Model file for the job. Use its own axes, mm. A direction names the side the tool comes from. Coordinates: 2 decimals unless noted, no trailing zeros. Order: outer loops, then holes, each group sorted by start corner. A loop starts at its lowest first (then second) coordinate and runs counter-clockwise, first axis right, second up. Notation, with made-up numbers: M 81,79.25 L 139,79.25 A18 cw 139,98.25 Z; hole C 59,19 d2. An arc over 180 degrees is marked long. Return JSON: item names as keys, results as strings.
```python
from build123d import *

# Parameters (mm, degrees)
SKETCH3_W                    = 130
SKETCH3_H                    = 107.95
BASE_FLANGE1_DEPTH           = 6.35
EDGE_FLANGE1_STRIP_W         = 26.8732
EDGE_FLANGE1_STRIP_H         = 6.35
EDGE_FLANGE1_STRIP_CUT_DEPTH = 107.95
EDGE_FLANGE1_DEPTH           = 107.95
EDGE_FLANGE1_PROFILE_W       = 107.95
EDGE_FLANGE1_PROFILE_H       = 210.4009
EDGE_FLANGE1_PROFILE_R       = 2.855235605
EDGE_FLANGE1_PROFILE_R_2     = 7.9375
EDGE_FLANGE1_FLAT_DEPTH      = 6.35
FILLET1_R                    = 25
SKETCH13_R                   = 2.6
FLANGE_COUPLING_HOLES_DEPTH  = 234.321909133
SKETCH15_R                   = 1.985
CUT_EXTRUDE1_DEPTH           = 234.321909133


# Sheet-metal steps are written as plain solids
with BuildPart() as part:
    # Sketch3 → Base-Flange1 (new body)
    with BuildSketch(Plane(origin=(0, 0, 0), x_dir=(1, 0, 0), z_dir=(0, 1, 0))):
        Rectangle(SKETCH3_W, SKETCH3_H)
    extrude(amount=-BASE_FLANGE1_DEPTH)

    # Edge-Flange1 strip (across the edge) → Edge-Flange1 strip cut (cut)
    with BuildSketch(Plane(origin=(65, -6.35, -53.975), x_dir=(-1, 0, 0), z_dir=(0, 0, 1))):
        with Locations((-6.35, -3.175)):
            Rectangle(EDGE_FLANGE1_STRIP_W, EDGE_FLANGE1_STRIP_H)
    edge_flange1_strip_cut = extrude(amount=EDGE_FLANGE1_STRIP_CUT_DEPTH, mode=Mode.SUBTRACT)

    # Edge-Flange1 bend section (across the edge) → Edge-Flange1 (add)
    with BuildSketch(Plane(origin=(65, -6.35, -53.975), x_dir=(-1, 0, 0), z_dir=(0, 0, 1))):
        with BuildLine():
            Line((0, 0.7366), (6.35, 0.7366))
            ThreePointArc((6.35, 0.7366), (6.565745145, 0.215745145), (7.0866, 0))
            Line((7.0866, 0), (7.0866, -6.35))
            ThreePointArc((7.0866, -6.35), (2.075617084, -4.274382916), (0, 0.7366))
        make_face()
    edge_flange1 = extrude(amount=EDGE_FLANGE1_DEPTH)

    # Edge-Flange1 profile (on flange) → Edge-Flange1 flat (add)
    with BuildSketch(Plane(origin=(65, -6.35, 0), x_dir=(0, 0, -1), z_dir=(-1, 0, 0))):
        with Locations((0, 105.93705)):
            Rectangle(EDGE_FLANGE1_PROFILE_W, EDGE_FLANGE1_PROFILE_H)
        with Locations((20, 177.8)):
            Circle(EDGE_FLANGE1_PROFILE_R, mode=Mode.SUBTRACT)
        with Locations((0, 177.8)):
            Circle(EDGE_FLANGE1_PROFILE_R_2, mode=Mode.SUBTRACT)
        with Locations((-20, 177.8)):
            Circle(EDGE_FLANGE1_PROFILE_R, mode=Mode.SUBTRACT)
    edge_flange1_flat = extrude(amount=EDGE_FLANGE1_FLAT_DEPTH)

    # Mirror1: Edge-Flange1 strip cut, Edge-Flange1, Edge-Flange1 flat across plane
    add(edge_flange1_strip_cut.mirror(Plane(origin=(0, 0, 0), x_dir=(0, 0, 1), z_dir=(1, 0, 0))), mode=Mode.SUBTRACT)
    add(edge_flange1.mirror(Plane(origin=(0, 0, 0), x_dir=(0, 0, 1), z_dir=(1, 0, 0))))
    add(edge_flange1_flat.mirror(Plane(origin=(0, 0, 0), x_dir=(0, 0, 1), z_dir=(1, 0, 0))))

    # Fillet1
    fillet1_edges = [part.edges().sort_by_distance(p)[0] for p in [
        (61.825, -217.4875, -53.975),
        (61.825, -217.4875, 53.975),
        (-61.825, -217.4875, 53.975),
        (-61.825, -217.4875, -53.975),
    ]]
    fillet(fillet1_edges, radius=FILLET1_R)

    # Sketch13 → Flange Coupling Holes (cut, through all)
    with BuildSketch(Plane(origin=(0, 0, 0), x_dir=(1, 0, 0), z_dir=(0, 1, 0))):
        with Locations(Location((-21.7, 0, 0), (0, 0, 270))):
            Circle(SKETCH13_R)
        with Locations(Location((-10.85, 18.792751262, 0), (0, 0, 270))):
            Circle(SKETCH13_R)
        with Locations(Location((10.85, 18.792751262, 0), (0, 0, 270))):
            Circle(SKETCH13_R)
        with Locations(Location((21.7, 0, 0), (0, 0, 270))):
            Circle(SKETCH13_R)
        with Locations(Location((10.85, -18.792751262, 0), (0, 0, 270))):
            Circle(SKETCH13_R)
        with Locations(Location((-10.85, -18.792751262, 0), (0, 0, 270))):
            Circle(SKETCH13_R)
    extrude(amount=-FLANGE_COUPLING_HOLES_DEPTH, mode=Mode.SUBTRACT)

    # Sketch15 → Cut-Extrude1 (cut, through all)
    with BuildSketch(Plane(origin=(0, 0, 0), x_dir=(1, 0, 0), z_dir=(0, 1, 0))):
        with Locations(Location((-44.845, 44.845, 0), (0, 0, 270))):
            Circle(SKETCH15_R)
        with Locations(Location((44.845, 44.845, 0), (0, 0, 270))):
            Circle(SKETCH15_R)
        with Locations(Location((44.845, -44.845, 0), (0, 0, 270))):
            Circle(SKETCH15_R)
        with Locations(Location((-44.845, -44.845, 0), (0, 0, 270))):
            Circle(SKETCH15_R)
    extrude(amount=-CUT_EXTRUDE1_DEPTH, mode=Mode.SUBTRACT)


solid = part.part
```
Item 1: Saw through at D-D (y = -115). Write the cut outline in (x, z) (3 decimals), and give its area (3 significant figures).
Check result:
{"outline": "M -65,-53.975 L -58.65,-53.975 L -58.65,53.975 L -65,53.975 Z; M 58.65,-53.975 L 65,-53.975 L 65,53.975 L 58.65,53.975 Z", "area": "1,370 mm2"}
Item 2: Pull direction Z, two halves, no side cores. Call faces 1 (the cylindrical face through (-62.87, -2.02, -0.76)), 2 (the cylindrical face through (61.781, -210.358, -46.457)), 3 (the cylindrical face through (61.87, -186.98, -19.63)), 4 (the cylindrical face through (61.87, -176.4, 1.72)): +Z half, -Z half, draft (parallel to the pull), parting line (faces both ways), or undercut.
Check result:
{"face 1": "draft", "face 2": "-Z half", "face 3": "undercut", "face 4": "undercut"}
Item 3: 3-axis set-ups, long thin cutter, end or side, ignore diameter. For faces 5 (the cylindrical face through (-61.87, -186.98, 20.37)), 6 (the flat face through (58.65, -114, 1)): which of +Z, -Z, +X, -X, +Y, -Y reach the whole face in a straight line?
Check result:
{"face 5": "+X, -X", "face 6": "+Z, -Z, -Y"}
Item 4: Drop flat-ended pins along their axis: pin 1 Ø3 at (x, z) = (42.5, -2) entering from -Y; pin 2 Ø7.5 at (y, z) = (-184.15, 20) entering from +X. Give the stop position or say it passes through.
Check result:
{"pin 1": "stops at y = -6.35", "pin 2": "stops at x = 65"}
Item 5: Saw through at C-C (z = 0). Write the cut outline in (x, y), and give its area (3 significant figures).
Check result:
{"outline": "M -65,-217.49 L -58.65,-217.49 L -58.65,-192.09 L -65,-192.09 Z; M -65,-176.21 L -58.65,-176.21 L -58.65,-7.09 A0.74 cw -57.91,-6.35 L -24.3,-6.35 L -24.3,0 L -57.91,0 A7.09 ccw -65,-7.09 Z; M -19.1,-6.35 L 19.1,-6.35 L 19.1,0 L -19.1,0 Z; M 24.3,-6.35 L 57.91,-6.35 A0.74 cw 58.65,-7.09 L 58.65,-176.21 L 65,-176.21 L 65,-7.09 A7.09 ccw 57.91,0 L 24.3,0 Z; M 58.65,-217.49 L 65,-217.49 L 65,-192.09 L 58.65,-192.09 Z", "area": "3,220 mm2"}
Item 6: Saw through at B-B (x = -21.7). Write the cut outline in (y, z) (3 decimals).
Check result:
{"outline": "M -6.35,-53.975 L 0,-53.975 L 0,-2.6 L -6.35,-2.6 Z; M -6.35,2.6 L 0,2.6 L 0,53.975 L -6.35,53.975 Z"}
Item 7: Saw through at A-A (y = -184.15). Count the separate pieces of the cut face and the enclosed holes in it, and give its area (3 significant figures).
Check result:
{"separate pieces": "8", "enclosed holes": "0", "area": "1,020 mm2"}
Item 8: Wall check: line 1 (X direction, y = -148.5, z = -10.5); line 2 (X direction, y = -2.75, z = 0); line 3 (Y direction, x = 36.5, z = 2). Give the ranges that are in metal, low to high.
Check result:
{"line 1": "x = -65 to -58.65, 58.65 to 65", "line 2": "x = -63.52 to -24.3, -19.1 to 19.1, 24.3 to 63.52", "line 3": "y = -6.35 to 0"}
